Geometry check sheet. Reference: the model listing, model coordinates, mm. A direction names the side the tool comes from. Give positions to 0.01 mm unless a question says otherwise; leave off trailing zeros. Write each loop counter-clockwise with the first axis right and the second up, starting at its lowest first coordinate (ties: lowest second). Pieces come first, ordered by that corner, then holes. Notation, with made-up numbers: M -10,73.25 L 9,73.25 A16 ccw 9,103.25 Z; hole C 50.5,59 d5. An arc over 180 degrees is marked long. Write each question's results on one line, items separated by ' | '.
```python
from build123d import *

# Parameters (mm, degrees)
SKETCH_1_W               = 82
SKETCH_1_H               = 82
SKETCH_1_R               = 35.5
EXTRUDE_1_DEPTH          = 245
SKETCH_2_W               = 82
SKETCH_2_H               = 82
EXTRUDE_2_DEPTH          = 27
SKETCH_3_W               = 8
SKETCH_3_H               = 20
CUT_EXTRUDE_1_DEPTH      = 245
SKETCH_4_R               = 4
CUT_EXTRUDE_2_DEPTH      = 20
FILLET_2_R               = 3
FILLET_3_R               = 3
FILLET_4_R               = 3
FILLET_5_R               = 3
SKETCH_5_R               = 1.05
CUT_EXTRUDE_3_DEPTH      = 10
EXTRUDE_START            = 0.2
SKETCH_6_R               = 1.05
EXTRUDE_3_DEPTH          = 0.2
CUT_EXTRUDE_5_REACH      = 263.591
SKETCH_7_W               = 20
SKETCH_7_H               = 65
CUT_EXTRUDE_6_REACH      = 263.591
SKETCH_8_W               = 41
SKETCH_8_H               = 20
SKETCH_9_R               = 1.2
CUT_EXTRUDE_7_DEPTH      = 12
CUT_EXTRUDE_8_DEPTH      = 262.591284258
CUT_EXTRUDE_8_DEPTH_BACK = 262.591284258
SKETCH_10_W              = 27
SKETCH_10_H              = 82


with BuildPart() as part:
    # 草圖1 → 填料-伸長1 (new body)
    with BuildSketch(Plane.XY):
        Rectangle(SKETCH_1_W, SKETCH_1_H)
        Circle(SKETCH_1_R, mode=Mode.SUBTRACT)
    extrude(amount=EXTRUDE_1_DEPTH)

    # 草圖2 → 填料-伸長2 (add)
    with BuildSketch(Plane(origin=(0, 0, 0), x_dir=(-1, 0, 0), z_dir=(0, 0, -1))):
        Rectangle(SKETCH_2_W, SKETCH_2_H)
    extrude(amount=EXTRUDE_2_DEPTH)

    # 草圖3 → 除料-伸長1 (cut)
    with BuildSketch(Plane.XY.offset(245)):
        with Locations((-37, 0)):
            Rectangle(SKETCH_3_W, SKETCH_3_H)
    extrude(amount=-CUT_EXTRUDE_1_DEPTH, mode=Mode.SUBTRACT)

    # 草圖4 → 除料-伸長2 (cut)
    with BuildSketch(Plane.XY.offset(245)):
        with Locations((-32.9, 33)):
            Circle(SKETCH_4_R)
        with Locations((33.1, 32.9)):
            Circle(SKETCH_4_R)
        with Locations((33, -33.1)):
            Circle(SKETCH_4_R)
        with Locations((-33, -33)):
            Circle(SKETCH_4_R)
    extrude(amount=-CUT_EXTRUDE_2_DEPTH, mode=Mode.SUBTRACT)

    # 圓角2
    fillet_2_edges = [part.edges().sort_by_distance(p)[0] for p in [
        (-36.9, 33, 225),
    ]]
    fillet(fillet_2_edges, radius=FILLET_2_R)

    # 圓角3
    fillet_3_edges = [part.edges().sort_by_distance(p)[0] for p in [
        (29.1, 32.9, 225),
    ]]
    fillet(fillet_3_edges, radius=FILLET_3_R)

    # 圓角4
    fillet_4_edges = [part.edges().sort_by_distance(p)[0] for p in [
        (-37, -33, 225),
    ]]
    fillet(fillet_4_edges, radius=FILLET_4_R)

    # 圓角5
    fillet_5_edges = [part.edges().sort_by_distance(p)[0] for p in [
        (29, -33.1, 225),
    ]]
    fillet(fillet_5_edges, radius=FILLET_5_R)

    # 草圖5 → 除料-伸長3 (cut)
    with BuildSketch(Plane(origin=(0, 41, 0), x_dir=(1, 0, 0), z_dir=(0, 1, 0))):
        with Locations(Location((-36.75, 22.75, 0), (0, 0, 270))):
            Circle(SKETCH_5_R)
        with Locations(Location((-36.75, 4.75, 0), (0, 0, 270))):
            Circle(SKETCH_5_R)
    extrude(amount=-CUT_EXTRUDE_3_DEPTH, mode=Mode.SUBTRACT)

    # 草圖6 → 填料-伸長3 (add)
    with BuildSketch(Plane(origin=(0, 35, 0), x_dir=(1, 0, 0), z_dir=(0, 1, 0)).offset(EXTRUDE_START)):
        with Locations(Location((-36.75, 22.75, 0), (0, 0, 270))):
            Circle(SKETCH_6_R)
        with Locations(Location((-36.75, 4.75, 0), (0, 0, 270))):
            Circle(SKETCH_6_R)
    extrude(amount=-EXTRUDE_3_DEPTH)

    # 草圖7 → 除料-伸長5 (cut, up to next)
    with BuildSketch(Plane(origin=(-41, 0, 0), x_dir=(0, 0, -1), z_dir=(1, 0, 0)), mode=Mode.PRIVATE) as cut_extrude_5_sk1:
        with Locations((17, -8.5)):
            Rectangle(SKETCH_7_W, SKETCH_7_H)
    cut_extrude_5_tool1 = extrude(cut_extrude_5_sk1.sketch, amount=CUT_EXTRUDE_5_REACH, mode=Mode.PRIVATE) & part.part
    add(cut_extrude_5_tool1.solids().sort_by_distance((-41, -8.5, -17))[0], mode=Mode.SUBTRACT)

    # 草圖8 → 除料-伸長6 (cut, up to next)
    with BuildSketch(Plane(origin=(0, 41, 0), x_dir=(1, 0, 0), z_dir=(0, 1, 0)), mode=Mode.PRIVATE) as cut_extrude_6_sk1:
        with Locations((20.5, 17)):
            Rectangle(SKETCH_8_W, SKETCH_8_H)
    cut_extrude_6_tool1 = extrude(cut_extrude_6_sk1.sketch, amount=-CUT_EXTRUDE_6_REACH, mode=Mode.PRIVATE) & part.part
    add(cut_extrude_6_tool1.solids().sort_by_distance((20.5, 41, -17))[0], mode=Mode.SUBTRACT)

    # 草圖9 → 除料-伸長7 (cut)
    with BuildSketch(Plane(origin=(0, 0, -7), x_dir=(-1, 0, 0), z_dir=(0, 0, -1))):
        with Locations((-33, 33)):
            Circle(SKETCH_9_R)
        with Locations((-33, -33)):
            Circle(SKETCH_9_R)
        with Locations((33, -33)):
            Circle(SKETCH_9_R)
        with Locations((36, 20)):
            Circle(SKETCH_9_R)
    extrude(amount=-CUT_EXTRUDE_7_DEPTH, mode=Mode.SUBTRACT)

    # 草圖10 → 除料-伸長8 (cut, two sides: drawn at the far end of the back side and taken through both)
    with BuildSketch(Plane.ZY.offset(41).offset(-CUT_EXTRUDE_8_DEPTH_BACK)):
        with Locations((-13.5, 0)):
            Rectangle(SKETCH_10_W, SKETCH_10_H)
    extrude(amount=CUT_EXTRUDE_8_DEPTH + CUT_EXTRUDE_8_DEPTH_BACK, mode=Mode.SUBTRACT)


solid = part.part
```
Q1. Material ranges on probe 1 along Y at (x, z) = (-32.9, 232); probe 2 along X at (y, z) = (13, 126); probe 3 along Y at (x, z) = (18, 146.5), recorded low to high. Write a range as [from, to].
Answer key:
probe 1: y = [-41, -37], [-29, -13.34], [13.34, 29], [37, 41] | probe 2: x = [-41, -33.03], [33.03, 41] | probe 3: y = [-41, -30.6], [30.6, 41]
Q2. Depth check by flat-ended pin: P1, Ø1.2, axis at x = -32.5, y = -33.5, coming from the -Z side; P2, Ø0.6, axis at x = -33, y = -33.5, coming from the +Z side; P3, Ø0.7, axis at x = 33, y = -32.5, coming from the -Z side; P4, Ø7, axis at x = 33, y = -33.1, coming from the +Z side. Enter the tip coordinate at first touch or a pass-through.
Answer key:
P1: stops at z = 0 | P2: stops at z = 225 | P3: stops at z = 5 | P4: stops at z = 226.34
Q3. Section check B-B (z = 140). Enter the section's corners in (x, y).
Answer key:
outline: M -41,-41 L 41,-41 L 41,41 L -41,41 L -41,10 L -34.06,10 A35.5 cw long -34.06,-10 L -41,-10 Z
Q4. Section check A-A (x = 0). Enter the section's corners in (y, z), then the cut area to 4 significant figures.
Answer key:
outline: M -41,0 L -35.5,0 L -35.5,245 L -41,245 Z; M 35.5,0 L 41,0 L 41,245 L 35.5,245 Z | area: 2,695 mm2
Q5. Section check D-D (y = 0). Enter the section's corners in (x, z).
Answer key:
outline: M 35.5,0 L 41,0 L 41,245 L 35.5,245 Z
Q6. Section check C-C (x = -11). Enter the section's corners in (y, z), then the cut area to 3 significant figures.
Answer key:
outline: M -41,0 L -33.75,0 L -33.75,245 L -41,245 Z; M 33.75,0 L 41,0 L 41,245 L 33.75,245 Z | area: 3,550 mm2
Q7. Release check for a two-part mould opening along Y. For faces 1 (the face through (41, -1, 124)), 2 (the face through (1, -41, 124)), 3 (the face through (29.9, 30.5, 236.6)), 4 (the face through (29.8, -35.5, 236.6)) record: released by +Y, released by -Y, zero draft, split by the parting line, or undercut.
Answer key:
face 1: zero draft | face 2: released by -Y | face 3: undercut | face 4: undercut
Q8. Access from +Z, -Z, +X, -X, +Y, -Y to the whole of each face (thin tool, end or side, straight path). Record for faces 5 (the face through (37, -1, 0)), 6 (the face through (-35.85, 35.7, 236.62)), 7 (the face through (-38, 10, 124)).
Answer key:
face 5: -Z, +X, -X, +Y, -Y | face 6: +Z | face 7: +Z, -Z, -X
